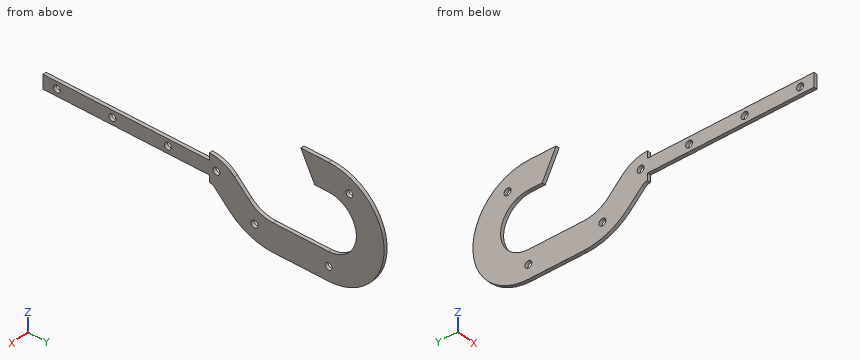
```python
from build123d import *

# Parameters (mm, degrees)
BOSS_EXTRUDE1_DEPTH = 3.175
SKETCH2_R           = 3.175
CUT_EXTRUDE1_DEPTH  = 4.175


with BuildPart() as part:
    # Sketch1 → Boss-Extrude1 (new body)
    with BuildSketch(Plane(origin=(0, 0, 0), x_dir=(0, 0, -1), z_dir=(1, 0, 0))):
        with BuildLine():
            Line((-50.8, 0), (-50.8, -25.4))
            Line((-50.8, -25.4), (-25.4, -12.7))
            Line((-25.4, -12.7), (-25.4, 0))
            ThreePointArc((-25.4, 0), (0, 25.4), (25.4, 0))
            Line((25.4, 0), (25.4, -50.8))
            ThreePointArc((25.4, -50.8), (22.983175157, -62.950198978), (16.100640303, -73.250640303))
            Line((16.100640303, -73.250640303), (3.130634922, -86.220645683))
            ThreePointArc((3.130634922, -86.220645683), (-3.886063261, -96.721876619), (-6.35, -109.108923092))
            Line((-6.35, -109.108923092), (0, -109.108923092))
            Line((0, -109.108923092), (0, -261.508923092))
            Line((0, -261.508923092), (12.7, -261.508923092))
            Line((12.7, -261.508923092), (12.7, -109.108923092))
            Line((12.7, -109.108923092), (19.05, -109.108923092))
            ThreePointArc((19.05, -109.108923092), (19.580476865, -106.442035801), (21.091147164, -104.181157925))
            Line((21.091147164, -104.181157925), (34.061152545, -91.211152545))
            ThreePointArc((34.061152545, -91.211152545), (46.449715283, -72.67035816), (50.8, -50.8))
            Line((50.8, -50.8), (50.8, 0))
            ThreePointArc((50.8, 0), (0, 50.8), (-50.8, 0))
        make_face()
    extrude(amount=BOSS_EXTRUDE1_DEPTH)

    # Sketch2 → Cut-Extrude1 (cut, through all)
    with BuildSketch(Plane(origin=(3.175, 0, 0), x_dir=(0, 0, -1), z_dir=(1, 0, 0))):
        with Locations((38.1, 0)):
            Circle(SKETCH2_R)
        with Locations((-32.995567884, 19.05)):
            Circle(SKETCH2_R)
        with Locations((34.71644522, -67.810278569)):
            Circle(SKETCH2_R)
        with Locations((6.35, -102.758923092)):
            Circle(SKETCH2_R)
        with Locations((6.35, -248.808923092)):
            Circle(SKETCH2_R)
        with Locations((6.35, -198.008923092)):
            Circle(SKETCH2_R)
        with Locations((6.35, -147.208923092)):
            Circle(SKETCH2_R)
    extrude(amount=-CUT_EXTRUDE1_DEPTH, mode=Mode.SUBTRACT)


solid = part.part
```
Read the model definition and answer for the solid it produces. Units are mm, in the model's axes. Give positions to 0.01 mm unless a question says otherwise; leave off trailing zeros. Write each loop counter-clockwise with the first axis right and the second up, starting at its lowest first coordinate (ties: lowest second). Pieces come first, ordered by that corner, then holes. Notation, with made-up numbers: (-15, -32) -> (36, -32) arc R10 cw to (36, -20) -> close; hole circle Ø7 at (20.25, 9). An arc over 180 degrees is marked (long way). Answer as a JSON object with one key per item and string values.
1) Flat-ended cylindrical pins translate along their axes: pin 1 Ø1.6 at (x, y) = (2, -199) entering from +Z; pin 2 Ø5.5 at (y, z) = (-147.21, -6.35) entering from +X; pin 3 Ø1 at (x, z) = (1, 1.5) entering from -Y. Find the tip coordinate at first contact, or state that the pin passes through.
Findings below:
{"pin 1": "stops at z = 0", "pin 2": "passes through", "pin 3": "stops at y = -109.11"}
2) Section D-D on y = -118.5 is taken. Write down the section's boundary in (x, z) (3 decimals).
Findings below:
{"outline": "(0, -12.7) -> (3.175, -12.7) -> (3.175, 0) -> (0, 0) -> close"}
3) Section B-B on z = -6.35 is taken. Write down the section's boundary in (x, y) (3 decimals).
Findings below:
{"outline": "(0, -261.509) -> (3.175, -261.509) -> (3.175, -251.984) -> (0, -251.984) -> close; (0, -245.634) -> (3.175, -245.634) -> (3.175, -201.184) -> (0, -201.184) -> close; (0, -194.834) -> (3.175, -194.834) -> (3.175, -150.384) -> (0, -150.384) -> close; (0, -144.034) -> (3.175, -144.034) -> (3.175, -105.934) -> (0, -105.934) -> close; (0, -99.584) -> (3.175, -99.584) -> (3.175, -83.001) -> (0, -83.001) -> close; (0, 24.593) -> (3.175, 24.593) -> (3.175, 50.402) -> (0, 50.402) -> close"}
4) Straight lines are drawn through the part: probe 1 along Y at (x, z) = (2.3, -6.35); probe 2 along Z at (x, y) = (0.4, -4.5); probe 3 along Z at (x, y) = (2.15, -163). For each, find the intervals that lie inside material, in ascending order. Write a range as from..to.
Findings below:
{"probe 1": "y = -261.51..-251.98, -245.63..-201.18, -194.83..-150.38, -144.03..-105.93, -99.58..-83, 24.59..50.4", "probe 2": "z = -50.8..-25.4, 25.4..50.8", "probe 3": "z = -12.7..0"}
5) Section C-C on x = 0.95 is taken. Write down the section's boundary in (y, z) (3 decimals), then the cut area to 3 significant figures.
Findings below:
{"outline": "(-261.509, -12.7) -> (-109.109, -12.7) -> (-109.109, -19.05) arc R6.969 cw to (-104.181, -21.091) -> (-91.211, -34.061) arc R57.15 ccw to (-50.8, -50.8) -> (0, -50.8) arc R50.8 ccw to (0, 50.8) -> (-25.4, 50.8) -> (-12.7, 25.4) -> (0, 25.4) arc R25.4 cw to (0, -25.4) -> (-50.8, -25.4) arc R31.75 cw to (-73.251, -16.101) -> (-86.221, -3.131) arc R32.369 ccw to (-109.109, 6.35) -> (-109.109, 0) -> (-261.509, 0) -> close; hole circle Ø6.35 at (-248.809, -6.35); hole circle Ø6.35 at (-198.009, -6.35); hole circle Ø6.35 at (-147.209, -6.35); hole circle Ø6.35 at (-102.759, -6.35); hole circle Ø6.35 at (-67.81, -34.716); hole circle Ø6.35 at (0, -38.1); hole circle Ø6.35 at (19.05, 32.996)", "area": "8,270 mm^2"}
6) Section A-A on y = 19.05 is taken. Write down the section's boundary in (x, z) (3 decimals), then the cut area to 3 significant figures.
Findings below:
{"outline": "(0, -47.093) -> (3.175, -47.093) -> (3.175, -16.801) -> (0, -16.801) -> close; (0, 16.801) -> (3.175, 16.801) -> (3.175, 29.821) -> (0, 29.821) -> close; (0, 36.171) -> (3.175, 36.171) -> (3.175, 47.093) -> (0, 47.093) -> close", "area": "172 mm^2"}
